Part print with two shaded views. Sizes in mm from the minimum x, y, z corner. A direction names the side the tool comes from. Round coordinates to 2 decimals unless told otherwise and drop trailing zeros. Loops run counter-clockwise (first coordinate to the right, second up) from the corner with the lowest first, then second, coordinate; pieces in that order, holes last. Notation, with made-up numbers: (64, 21) -> (72, 21) arc R23 cw to (72, 52) -> close; hole circle Ø3 at (19, 42.25). An arc over 180 degrees is marked (long way). Answer as a JSON object with one key per item and string values. Group by question number.
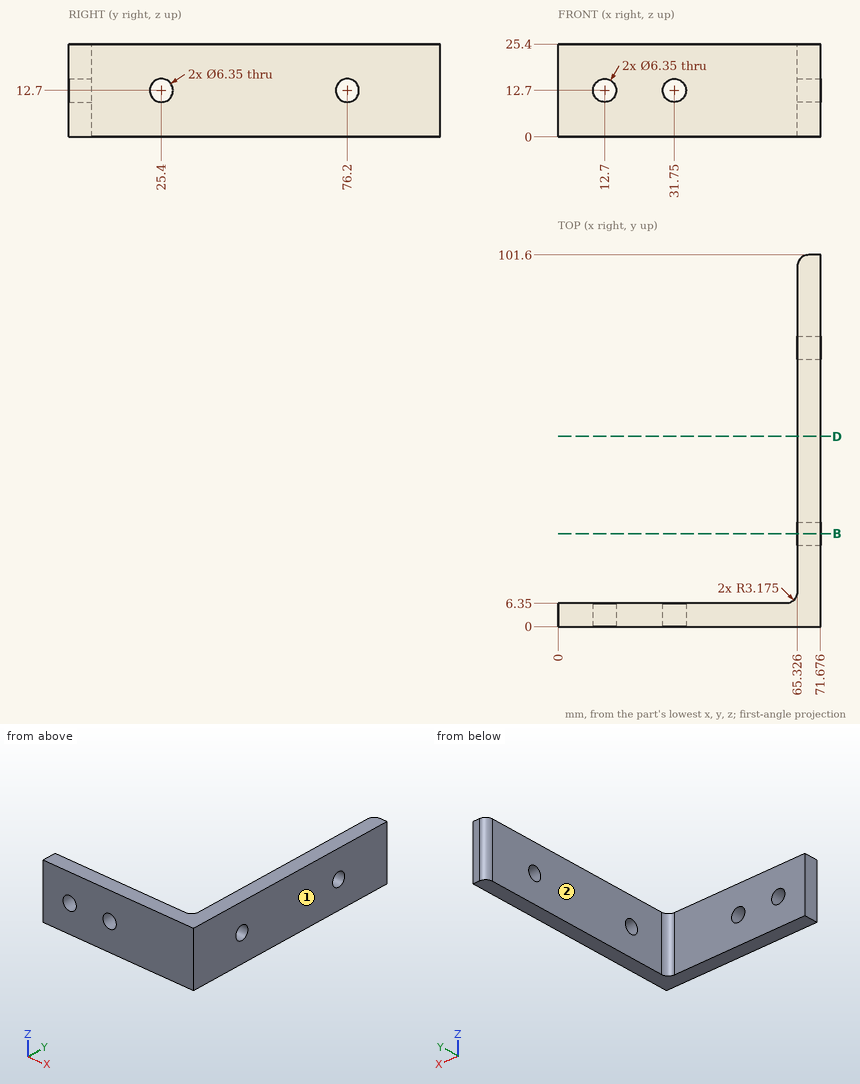
Item 1: Which spindle directions (+Z, -Z, +X, -X, +Y, -Y) get a long thin tool onto all of the face, cutting with end or side? Do the marked faces 1 and 2. Say none if no direction does.
Item 2: Drill centre lines: line 1 (Y direction, x = 69, z = 12.7) (1 decimal); line 2 (Y direction, x = 67, z = 12.7) (1 decimal); line 3 (Z direction, x = 67, y = 25). Where is each one in solid material? Low to high.
Item 3: Drop flat-ended pins along their axis: pin 1 Ø5.5 at (x, z) = (12.7, 12.7) entering from -Y; pin 2 Ø12.5 at (x, z) = (23.5, 8) entering from +Y; pin 3 Ø1 at (y, z) = (85, 7.5) entering from -X. Give the stop position or say it passes through.
Item 4: Band-saw the part on D-D, the plane y = 52. List the corners of the cut face in (x, z), plus the area to 3 significant figures.
Item 5: Band-saw the part on B-B, the plane y = 25.4. List the corners of the cut face in (x, z) (1 decimal).
Entries:
{
 "1": {"face 1": "+Z, -Z, +X, +Y, -Y", "face 2": "+Z, -Z, -X, +Y"},
 "2": {"line 1": "0 to 22.2, 28.6 to 73, 79.4 to 101.6", "line 2": "0 to 22.2, 28.6 to 73, 79.4 to 101.2", "line 3": "0 to 9.55, 15.85 to 25.4"},
 "3": {"pin 1": "through", "pin 2": "y = 6.35", "pin 3": "x = 65.33"},
 "4": {"outline": "(65.33, 0) -> (71.68, 0) -> (71.68, 25.4) -> (65.33, 25.4) -> close", "area": "161 mm²"},
 "5": {"outline": "(65.3, 0) -> (71.7, 0) -> (71.7, 9.5) -> (65.3, 9.5) -> close; (65.3, 15.9) -> (71.7, 15.9) -> (71.7, 25.4) -> (65.3, 25.4) -> close"}
}
